from build123d import *

# Parameters (mm, degrees)
SKETCH2_W               = 550
SKETCH2_H               = 450
BOSS_EXTRUDE1_DEPTH     = 100
SKETCH3_W               = 50
SKETCH3_H               = 100
BOSS_EXTRUDE2_DEPTH     = 125
MIRROR2_COPY_1_SKETCH_W = 50
MIRROR2_COPY_1_SKETCH_H = 100
MIRROR2_COPY_1_DEPTH    = 125
SKETCH4_R               = 31
CUT_EXTRUDE1_DEPTH      = 16
MIRROR4_COPY_1_SKETCH_R = 31
MIRROR4_COPY_1_DEPTH    = 16
FILLET4_R               = 10


with BuildPart() as part:
    # Sketch2 → Boss-Extrude1 (new body)
    with BuildSketch(Plane(origin=(0, 0, 0), x_dir=(1, 0, 0), z_dir=(0, 1, 0))):
        with Locations((111.087570621, 17.973163842)):
            Rectangle(SKETCH2_W, SKETCH2_H)
    boss_extrude1 = extrude(amount=BOSS_EXTRUDE1_DEPTH)

    # Sketch3 → Boss-Extrude2 (add)
    with BuildSketch(Plane.ZY.offset(163.912429379)):
        with Locations((-217.973163842, 50)):
            Rectangle(SKETCH3_W, SKETCH3_H)
    boss_extrude2 = extrude(amount=BOSS_EXTRUDE2_DEPTH)

    # Mirror1: Boss-Extrude2 across plane
    add(boss_extrude2.mirror(Plane(origin=(0, 0, -17.973163842), x_dir=(1, 0, 0), z_dir=(0, 0, -1))))

    # Mirror2: Boss-Extrude1, Boss-Extrude2 across plane
    add(boss_extrude1.mirror(Plane(origin=(111.087570621, 0, 0), x_dir=(0, 0, 1), z_dir=(1, 0, 0))))
    add(boss_extrude2.mirror(Plane(origin=(111.087570621, 0, 0), x_dir=(0, 0, 1), z_dir=(1, 0, 0))))

    # Mirror2 copy 1 sketch → Mirror2 copy 1 (add)
    with BuildSketch(Plane(origin=(386.087570621, 0, -35.946327684), x_dir=(0, 0, -1), z_dir=(1, 0, 0))):
        with Locations((-217.973163842, 50)):
            Rectangle(MIRROR2_COPY_1_SKETCH_W, MIRROR2_COPY_1_SKETCH_H)
    extrude(amount=MIRROR2_COPY_1_DEPTH)

    # Sketch4 → Cut-Extrude1 (cut)
    with BuildSketch(Plane(origin=(0, 0, 157.026836158), x_dir=(-1, 0, 0), z_dir=(0, 0, -1))):
        with Locations((-448.587570621, 50)):
            Circle(SKETCH4_R)
    cut_extrude1 = extrude(amount=-CUT_EXTRUDE1_DEPTH, mode=Mode.SUBTRACT)

    # Mirror3: Cut-Extrude1 across plane
    add(cut_extrude1.mirror(Plane(origin=(0, 0, -17.973163842), x_dir=(1, 0, 0), z_dir=(0, 0, -1))), mode=Mode.SUBTRACT)

    # Mirror4: Cut-Extrude1 across plane
    add(cut_extrude1.mirror(Plane(origin=(111.087570621, 0, 0), x_dir=(0, 0, 1), z_dir=(1, 0, 0))), mode=Mode.SUBTRACT)

    # Mirror4 copy 1 sketch → Mirror4 copy 1 (cut)
    with BuildSketch(Plane(origin=(222.175141243, 0, -192.973163842), x_dir=(1, 0, 0), z_dir=(0, 0, 1))):
        with Locations((-448.587570621, 50)):
            Circle(MIRROR4_COPY_1_SKETCH_R)
    extrude(amount=-MIRROR4_COPY_1_DEPTH, mode=Mode.SUBTRACT)

    # Fillet4
    fillet4_edges = [part.edges().sort_by_distance(p)[0] for p in [
        (386.087570621, 0, -17.973163842),
        (386.087570621, 100, -17.973163842),
        (448.587570621, 0, 157.026836158),
        (448.587570621, 100, 157.026836158),
        (511.087570621, 0, 182.026836158),
        (511.087570621, 100, 182.026836158),
        (111.087570621, 100, -242.973163842),
        (-163.912429379, 0, -17.973163842),
        (-163.912429379, 100, -17.973163842),
        (-226.412429379, 0, -192.973163842),
        (-226.412429379, 100, -192.973163842),
        (-288.912429379, 0, -217.973163842),
        (-288.912429379, 100, -217.973163842),
        (-288.912429379, 100, 182.026836158),
        (-226.412429379, 100, 157.026836158),
        (-288.912429379, 0, 182.026836158),
        (-226.412429379, 0, 157.026836158),
        (111.087570621, 0, -242.973163842),
        (111.087570621, 0, 207.026836158),
        (511.087570621, 100, -217.973163842),
        (111.087570621, 100, 207.026836158),
        (448.587570621, 100, -192.973163842),
        (511.087570621, 0, -217.973163842),
        (448.587570621, 0, -192.973163842),
    ]]
    fillet(fillet4_edges, radius=FILLET4_R)


solid = part.part
Work out the finished part from the listing and answer in its coordinate system (mm). A direction names the side the tool comes from. Coordinates: 2 decimals unless noted, no trailing zeros. Write each loop counter-clockwise with the first axis right and the second up, starting at its lowest first coordinate (ties: lowest second). Pieces come first, ordered by that corner, then holes.
1. Consider line 1 along Z through (x, y) = (443, 82.5); line 2 along X through (y, z) = (40, -195); line 3 along X through (y, z) = (32, -196). Determine where each line is inside the solid, lowest interval first.
Results list:
line 1: z = -242.97 to -192.97, 157.03 to 207.03
line 2: x = -288.91 to -255.76, -197.07 to 419.24, 477.93 to 511.09
line 3: x = -288.91 to -251.65, -201.17 to 423.35, 473.83 to 511.09
2. For faces 1 (the flat face through (511.088, 51, -218)), 2 (the flat face through (-227, 50, -208.973)), 3 (the flat face through (420, 67, 157.027)), 4 (the flat face through (-253, 67, 157.027)), determine the directions among +Z, -Z, +X, -X, +Y, -Y from which every point of the face is accessible in a straight line to the end or side of a thin tool.
Results list:
face 1: +Z, -Z, +X, +Y, -Y
face 2: none
face 3: +X, +Y, -Y
face 4: -X, +Y, -Y
3. The part is cut by section A-A, the plane x = 409. Write down the section's boundary in (y, z).
Results list:
outline: (0, -232.97) arc R10 ccw to (10, -242.97) - (90, -242.97) arc R10 ccw to (100, -232.97) - (100, -202.97) arc R10 ccw to (90, -192.97) - (10, -192.97) arc R10 ccw to (0, -202.97) - close; (0, 167.03) arc R10 ccw to (10, 157.03) - (90, 157.03) arc R10 ccw to (100, 167.03) - (100, 197.03) arc R10 ccw to (90, 207.03) - (10, 207.03) arc R10 ccw to (0, 197.03) - close
4. Flat-ended cylindrical pins translate along their axes: pin 1 (24 mm diameter, centred on y = 44.5, z = -92.5, fed in from -X); pin 2 (4 mm diameter, centred on y = 39.5, z = -31.5, fed in from +X). Find the tip coordinate at first contact, or state that the pin passes through.
Results list:
pin 1: stops at x = -163.91
pin 2: stops at x = 386.09
5. For a pull along Z with two mould halves and no side action, classify faces 5 (the flat face through (105, 49, 207.027)), 6 (the flat face through (105, 49, -242.973)), 7 (the cylindrical face through (419.02, 59.31, -200.86)), 8 (the flat face through (106, 100, -15)) as +Z half, -Z half, draft (parallel to the pull), parting line (faces both ways), or undercut.
Results list:
face 5: +Z half
face 6: -Z half
face 7: undercut
face 8: draft
6. The part is cut by section B-B, the plane y = 50. Write down the section's boundary in (x, z), and give its area (3 significant figures).
Results list:
outline: (-288.91, -242.97) - (511.09, -242.97) - (511.09, -192.97) - (479.59, -192.97) - (479.59, -208.97) - (417.59, -208.97) - (417.59, -192.97) - (386.09, -192.97) - (386.09, 157.03) - (417.59, 157.03) - (417.59, 173.03) - (479.59, 173.03) - (479.59, 157.03) - (511.09, 157.03) - (511.09, 207.03) - (-288.91, 207.03) - (-288.91, 157.03) - (-257.41, 157.03) - (-257.41, 173.03) - (-195.41, 173.03) - (-195.41, 157.03) - (-163.91, 157.03) - (-163.91, -192.97) - (-195.41, -192.97) - (-195.41, -208.97) - (-257.41, -208.97) - (-257.41, -192.97) - (-288.91, -192.97) - close
area: 269,000 mm2
7. The part is cut by section C-C, the plane z = -84.5. Write down the section's boundary in (x, y).
Results list:
outline: (-163.91, 10) arc R10 ccw to (-153.91, 0) - (376.09, 0) arc R10 ccw to (386.09, 10) - (386.09, 90) arc R10 ccw to (376.09, 100) - (-153.91, 100) arc R10 ccw to (-163.91, 90) - close
